Check sheet for the drawn part. Datum: minimum x, y, z corner. Units: mm. A direction names the side the tool comes from. Coordinates: 2 decimals unless noted, no trailing zeros. Write each loop counter-clockwise with the first axis right and the second up, starting at its lowest first coordinate (ties: lowest second). Pieces come first, ordered by that corner, then holes. Notation, with made-up numbers: (17, 74.5) - (26, 74.5) arc R36 cw to (26, 109.5) - close; hole circle Ø6 at (22, -11). An arc over 180 degrees is marked (long way). Use CSV: the item, a comma, the result in double quotes. Start each with the question number.
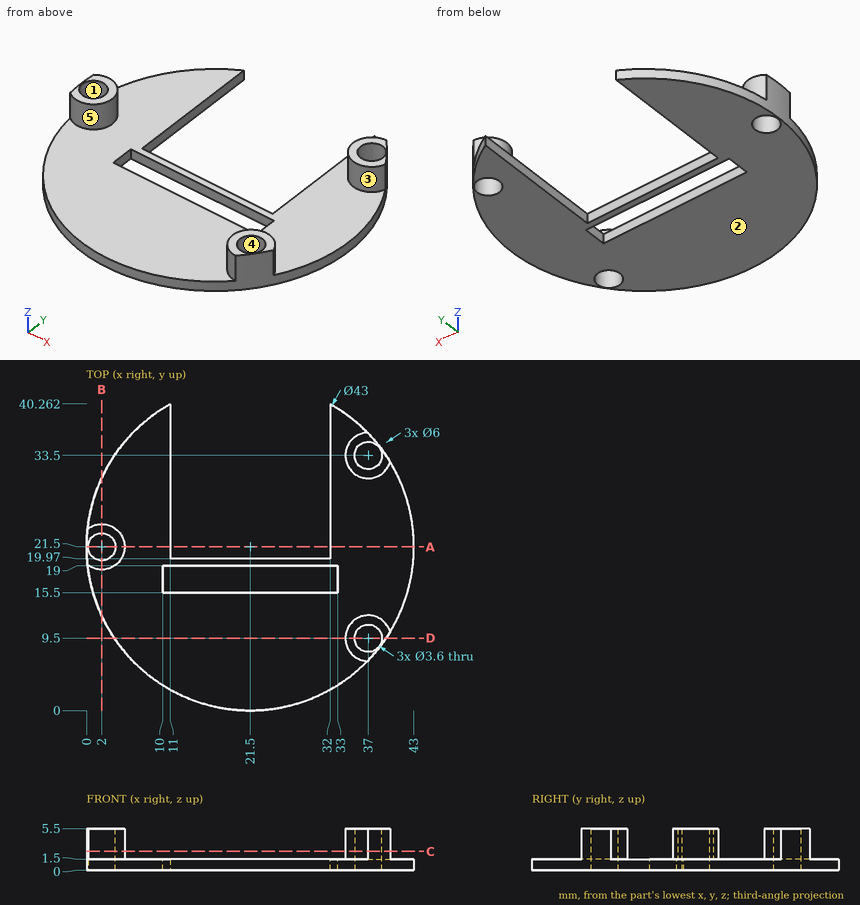
Q1. Cross-section at D-D (y = 9.5). Record the cut outline in (x, z).
Q2. Release check for a two-part mould opening along X. For the marked faces 1, 2 and 3 record: released by +X, released by -X, zero draft, split by the parting line, or undercut.
Q3. Cross-section at A-A (y = 21.5). Record the cut outline in (x, z), plus the area to 3 significant figures.
Q4. Cross-section at B-B (x = 2). Record the cut outline in (y, z) (1 decimal).
Q5. Cross-section at C-C (z = 2.5). Record the cut outline in (x, y) (1 decimal).
Q6. Scan lines: line 1 along Y through (x, z) = (2, 1.7); line 2 along Y through (x, z) = (18.5, 1); line 3 along X through (y, z) = (21.5, 1.4). Record each from-to range of solid material in increasing order. Write a range as from..to.
Q7. Tool access check on the marked faces 4 and 5. Record the directions out of +Z, -Z, +X, -X, +Y, -Y that give a thin tool (end or side, any length) a straight path to the whole face; none if there is none.
Q8. Gauge pin test, flat ends, axial feed: pin 1 (1.2 mm diameter, centred on x = 19.5, z = 0.5, fed in from -Y); pin 2 (0.8 mm diameter, centred on y = 30.5, z = 1, fed in from -X) (1 decimal); pin 3 (2 mm diameter, centred on y = 28.5, z = 1, fed in from +X); pin 4 (12 mm diameter, centred on x = 17.5, y = 35, fed in from +Z). Record the tip position at first contact, or that the pin passes through.
Reply:
1,outline,"(3.66, 0) - (35.2, 0) - (35.2, 5.5) - (34, 5.5) - (34, 1.5) - (3.66, 1.5) - close; (38.8, 0) - (39.34, 0) - (39.34, 5.5) - (38.8, 5.5) - close"
2,face 1,"undercut"
2,face 2,"zero draft"
2,face 3,"split by the parting line"
3,outline,"(0, 0) - (0.2, 0) - (0.2, 5.5) - (0, 5.5) - close; (3.8, 0) - (11, 0) - (11, 1.5) - (5, 1.5) - (5, 5.5) - (3.8, 5.5) - close; (32, 0) - (43, 0) - (43, 1.5) - (32, 1.5) - close"
3,area,"33.2 mm^2"
4,outline,"(12.4, 0) - (19.7, 0) - (19.7, 5.5) - (18.5, 5.5) - (18.5, 1.5) - (12.4, 1.5) - close; (23.3, 0) - (30.6, 0) - (30.6, 1.5) - (24.5, 1.5) - (24.5, 5.5) - (23.3, 5.5) - close"
5,outline,"(0.1, 19.2) arc R3 ccw (long way) to (0.1, 23.8) arc R21.5 ccw to start; (36.9, 6.5) arc R21.5 ccw to (39.9, 10.3) arc R3 ccw (long way) to start; (36.9, 36.5) arc R3 ccw (long way) to (39.9, 32.7) arc R21.5 ccw to start; hole circle Ø3.6 at (2, 21.5); hole circle Ø3.6 at (37, 9.5); hole circle Ø3.6 at (37, 33.5)"
6,line 1,"18.5..19.7, 23.3..24.5"
6,line 2,"0.21..15.5, 19..19.97"
6,line 3,"0..0.2, 3.8..11, 32..43"
7,face 4,"+Z, -Z"
7,face 5,"+Z"
8,pin 1,"y = 0.05"
8,pin 2,"x = 1.8"
8,pin 3,"x = 42.15"
8,pin 4,"through"
